from build123d import *

# Parameters (mm, degrees)
SCHIZZO1_R                   = 12
ESTRUSIONE_ESTRUSIONE1_DEPTH = 5
SCHIZZO3_R                   = 8.6
TAGLIO_ESTRUSIONE1_DEPTH     = 18.691806013
SMUSSO1_SIZE                 = 0.5
SMUSSO2_SIZE                 = 0.5


with BuildPart() as part:
    # Schizzo1 → Estrusione-Estrusione1 (new body)
    with BuildSketch(Plane.XY):
        Circle(SCHIZZO1_R)
    extrude(amount=ESTRUSIONE_ESTRUSIONE1_DEPTH)

    # Schizzo3 → Taglio-Estrusione1 (cut, through all)
    with BuildSketch(Plane.XY.offset(5)):
        Circle(SCHIZZO3_R)
    extrude(amount=-TAGLIO_ESTRUSIONE1_DEPTH, mode=Mode.SUBTRACT)

    # Smusso1
    smusso1_edges = [part.edges().sort_by_distance(p)[0] for p in [
        (-12, 0, 5),
    ]]
    chamfer(smusso1_edges, length=SMUSSO1_SIZE)

    # Smusso2
    smusso2_edges = [part.edges().sort_by_distance(p)[0] for p in [
        (-12, 0, 0),
    ]]
    chamfer(smusso2_edges, length=SMUSSO2_SIZE)


solid = part.part
The model under review builds one solid part; all positions refer to its coordinate system, in mm. Round coordinates to 2 decimals unless told otherwise and drop trailing zeros. Loops run counter-clockwise (first coordinate to the right, second up) from the corner with the lowest first, then second, coordinate; pieces in that order, holes last. Notation, with made-up numbers: M 72.25,-33 L 77.25,-33 A13 cw 77.25,-29 Z; hole C 28.5,44 d1. An arc over 180 degrees is marked long. Answer as a JSON object with one key per item and string values.
Item 1: The part is to be moulded in two halves that separate along X. For faces 1 (the face through (-8.59, 0.38, 2.54)), 2 (the face through (4, -8, 0)), 3 (the face through (-11.99, 0.53, 2.47)), say which applies: +X half, -X half, draft (parallel to the pull), parting line (faces both ways), or undercut.
Check sheet entries:
{"face 1": "undercut", "face 2": "draft", "face 3": "parting line"}
Item 2: We need section A-A, the plane y = 0. State the section outline as (x, z) points, and give its area (3 significant figures).
Check sheet entries:
{"outline": "M -12,0.5 L -11.5,0 L -8.6,0 L -8.6,5 L -11.5,5 L -12,4.5 Z; M 8.6,0 L 11.5,0 L 12,0.5 L 12,4.5 L 11.5,5 L 8.6,5 Z", "area": "33.5 mm2"}
Item 3: Clearance check with flat-ended pins moving along their axes: P1, Ø3, axis at x = 2, z = 2.5, coming from the -Y side; P2, Ø3, axis at x = -2, z = 4, coming from the +Y side; P3, Ø2, axis at x = -3.5, z = 3, coming from the +Y side. State where each tip first meets the part, or that it passes through.
Check sheet entries:
{"P1": "y = -11.99", "P2": "y = 11.99", "P3": "y = 11.74"}
Item 4: We need section C-C, the plane z = 2.9. State the section outline as (x, y) points.
Check sheet entries:
{"outline": "C 0,0 d24; hole C 0,0 d17.2"}
Item 5: For line 1 along Y through (x, z) = (-0.25, 3.55); line 2 along Y through (x, z) = (2, 1.1); line 3 along X through (y, z) = (1.5, 1.3), list the stretches that pass through material, from the lowest coordinate up.
Check sheet entries:
{"line 1": "-12 to -8.6, 8.6 to 12", "line 2": "-11.83 to -8.36, 8.36 to 11.83", "line 3": "-11.91 to -8.47, 8.47 to 11.91"}
